Autodesk Inventor part; units mm, degrees
ref_plane "YZ Plane" through (0, 0, 0) normal (1, 0, 0) x (0, 1, 0)
ref_plane "XZ Plane" through (0, 0, 0) normal (0, 1, 0) x (-1, 0, 0)
ref_plane "XY Plane" through (0, 0, 0) normal (0, 0, 1) x (1, 0, 0)
sketch "Sketch1" plane through (0, 0, 0) normal (0, 0, 1) x (1, 0, 0)
  line L0 (0, 0) -> (3.8, 0)
  line L1 (3.8, 0) -> (3.8, 17) construction
  line L2 (3.8, 17) -> (0, 17)
  line L3 (0, 17) -> (0, 0) construction
  line L4 (3.8, 17) -> (3.8, 11.325)
  line L5 (3.8, 0) -> (3.8, 5.675)
  line L6 (3.8, 8.5) -> (16.8, 8.5) construction
  line L7 (16.8, 10.45) -> (16.8, 6.55) construction
  line L8 (3.8, 5.675) -> (18.8, 6.6846)
  line L9 (3.8, 11.325) -> (18.8, 10.3154)
  line L10 (18.8, 10.3154) -> (18.8, 6.6846)
  line L11 (0, 17) -> (0, 12)
  line L12 (0, 0) -> (0, 5)
  line L13 (0, 8.5) -> (-15, 8.5) construction
  line L14 (-15, 10.5) -> (-15, 6.5) construction
  line L15 (0, 12) -> (-16, 10.4)
  line L16 (0, 5) -> (-16, 6.6)
  line L17 (-16, 10.4) -> (-16, 6.6)
  dimension "d0" = 3.8
  dimension "d1" = 17
  dimension "d2" = 5.675
  dimension "d3" = 5.675
  dimension "d4" = 13
  dimension "d5" = 3.9
  dimension "d8" = 15
  dimension "d9" = 15
  dimension "d10" = 5
  dimension "d11" = 5
  dimension "d12" = 15
  dimension "d13" = 4
  dimension "d14" = 16
  dimension "d15" = 16
  dimension "d75" = 7.701
extrude "Horn_Body" add sketch "Sketch1" along normal blind 2
fillet "Fillet1" radius 1.9 4 edges at (3.8, 17, 1) (0, 17, 1) (0, 0, 1) (3.8, 0, 1)
fillet "Fillet2" radius 1.9 2 edges at (18.8, 6.6846, 1) (18.8, 10.3154, 1)
fillet "Fillet3" radius 2 2 edges at (-16, 10.4, 1) (-16, 6.6, 1)
sketch "Sketch2" plane through (0, 0, 0) normal (0, 0, -1) x (-1, 0, 0)
  circle A0 centre (-1.9, 8.5) radius 3.55
  line L0 (18.55, 8.5) -> (-27.4875, 8.5) construction
  line L1 (16, 8.59) -> (16, 8.41)
  line L2 (-1.9, 22.225) -> (-1.9, -4.7625) construction
  line L3 (-3.8, 11.325) -> (-3.8, 15.1)
  line L4 (0, 15.1) -> (0, 12)
  point P0 (0, 0)
  point P1 (16, 8.5)
  dimension "d21" = 7.1
  dimension "d22" = 3.8
  dimension "d23" = 1.9
extrude "Shaft_Connector" add sketch "Sketch2" along normal blind 2.7
sketch "Sketch3" plane through (1.9, 8.5, -2.7) normal (0, 0, -1) x (-1, 0, 0)
  circle A0 centre (0, 0) radius 2.25
  point P0 (1.9, -8.5)
  dimension "d26" = 4.5
extrude "Shaft_Opening" cut sketch "Sketch3" against normal blind 2
sketch "Sketch4" plane through (1.9, 8.5, -0.7) normal (0, 0, -1) x (-1, 0, 0)
  circle A0 centre (0, 0) radius 1.25
  point P0 (1.9, -8.5)
  dimension "d29" = 2.5
extrude "Opening_Horn_FixationScrew" cut sketch "Sketch4" against normal up to surface (2.7 mm away)
sketch "Sketch6" plane through (0, 0, 2) normal (0, 0, 1) x (1, 0, 0)
  line L0 (-18.55, 8.5) -> (21.1375, 8.5) construction
  line L1 (-16, 8.59) -> (-16, 8.41)
  line L2 (1.9, 19.05) -> (1.9, -2.3164) construction
  line L3 (3.8, 11.325) -> (3.8, 15.1)
  line L4 (0, 15.1) -> (0, 12)
  circle A0 centre (-11.1, 8.54) radius 0.25
  circle A1 centre (-9.1, 8.5) radius 0.25
  circle A2 centre (-7.1, 8.5) radius 0.25
  circle A3 centre (-3.1, 8.5) radius 0.25
  circle A4 centre (-5.1, 8.5) radius 0.25
  circle A5 centre (-13.1, 8.5) radius 0.25
  circle A6 centre (-15.1, 8.5) radius 0.25
  circle A7 centre (6.9, 8.5) radius 0.25
  circle A8 centre (8.9, 8.5) radius 0.25
  circle A9 centre (10.9, 8.5) radius 0.25
  circle A10 centre (12.9, 8.5) radius 0.25
  circle A11 centre (14.9, 8.5) radius 0.25
  circle A12 centre (16.9, 8.5) radius 0.25
  circle A13 centre (1.9, 13.5) radius 0.25
  circle A14 centre (1.9, 15.5) radius 0.25
  circle A15 centre (1.9, 3.5) radius 0.25
  circle A16 centre (1.9, 1.5) radius 0.25
  point P0 (0, 0)
  point P1 (-16, 8.5)
  dimension "d35" = 3.8
  dimension "d36" = 1.9
  dimension "d37" = 0.5
  dimension "d38" = 0.5
  dimension "d39" = 0.5
  dimension "d41" = 0.5
  dimension "d42" = 0.5
  dimension "d43" = 5
  dimension "d44" = 2
  dimension "d46" = 2
  dimension "d47" = 2
  dimension "d48" = 2
  dimension "d49" = 0.5
  dimension "d50" = 0.5
  dimension "d51" = 2
  dimension "d52" = 2
  dimension "d53" = 0.5
  dimension "d54" = 0.5
  dimension "d55" = 0.5
  dimension "d56" = 0.5
  dimension "d57" = 0.5
  dimension "d58" = 5
  dimension "d59" = 2
  dimension "d60" = 2
  dimension "d61" = 2
  dimension "d62" = 2
  dimension "d63" = 0.5
  dimension "d64" = 2
  dimension "d65" = 0.5
  dimension "d66" = 0.5
  dimension "d67" = 0.5
  dimension "d68" = 0.5
  dimension "d69" = 5
  dimension "d70" = 2
  dimension "d71" = 5
  dimension "d72" = 2
extrude "Connection_Holes" cut sketch "Sketch6" against normal up to surface (2 mm away)
sketch "Sketch8" plane through (0, 0, 2) normal (0, 0, 1) x (1, 0, 0)
  circle A0 centre (1.9, 8.5) radius 1.25
  circle A1 centre (1.9, 8.5) radius 2.5
  circle A2 centre (1.9, 8.5) radius 3.1
  point P0 (0, 0)
  dimension "d80" = 5
  dimension "d81" = 6.2
extrude "Centering_RIng" add sketch "Sketch8" along normal blind 1 contours A2
equation "\"d14\" = d15"
equation "\"d23\" = 0.5 * d22"
equation "\"d36\" = 0.5 * d35"
properties part number "Servo_Horn_Cross_TGY"
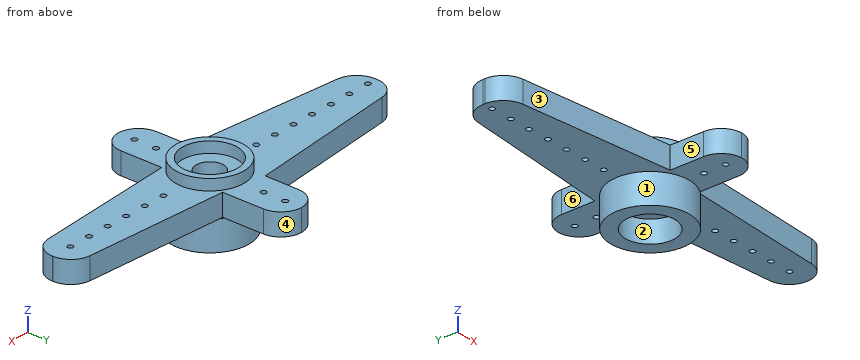
Geometry: final body of the model. Coordinates: model frame, mm. Face numbers are marked on the shaded views. A direction names the side the tool comes from. Coordinates: 2 decimals unless noted, no trailing zeros. Order: outer loops, then holes, each group sorted by start corner. A loop starts at its lowest first (then second) coordinate and runs counter-clockwise, first axis right, second up. Notation, with made-up numbers: (-34.5, 46) -> (1.5, 46) arc R35 ccw to (1.5, 78) -> close; hole circle Ø10 at (-24.5, 37.25). An arc over 180 degrees is marked (long way). Use CSV: the item, a comma, the result in double quotes.
1) Pin query (flat end, axial travel): pin 1 Ø5 at (x, y) = (1, 8) entering from -Z; pin 2 Ø1.6 at (y, z) = (13.5, 0.5) entering from -X; pin 3 Ø3 at (x, y) = (12, 7.5) entering from -Z; pin 4 Ø1 at (y, z) = (4.5, 1) entering from +X. Return the tip coordinate at first contact, or that it passes through.
Findings:
pin 1,"stops at z = -2.7"
pin 2,"stops at x = 0"
pin 3,"stops at z = 0"
pin 4,"stops at x = 3.8"
2) Line query: line 1 (Y direction, x = 1.9, z = 1.6); line 2 (Y direction, x = 16.9, z = 1); line 3 (Z direction, x = 4, y = 9.75). Output: solid intervals per line, ascending.
Findings:
line 1,"y = 0 to 1.25, 1.75 to 3.25, 3.75 to 7.25, 9.75 to 13.25, 13.75 to 15.25, 15.75 to 17"
line 2,"y = 6.56 to 8.25, 8.75 to 10.44"
line 3,"z = -2.7 to 2"
3) Access query for the marked faces 4, 5 and 6. Directions: +Z, -Z, +X, -X, +Y, -Y. A direction counts if a zero-diameter tool reaches every point of the face in a straight line with its end or side. Return the directions, or none.
Findings:
face 4,"+Z, -Z, +X, +Y"
face 5,"+Z, -Z, -X, -Y"
face 6,"+Z, -Z, -X, +Y"
4) Mould query, pull axis X, two halves, no side actions, for the marked faces 1, 2 and 3. Classes: +X half, -X half, draft (parallel to the pull), parting line (faces both ways), or undercut.
Findings:
face 1,"parting line"
face 2,"undercut"
face 3,"-X half"
5) Section C-C on x = 14. Output: boundary loops of the cut face in (y, z).
Findings:
outline,"(6.36, 0) -> (10.64, 0) -> (10.64, 2) -> (6.36, 2) -> close"
6) Section B-B on x = -4.5. Output: boundary loops of the cut face in (y, z), then the cut area to 3 significant figures.
Findings:
outline,"(5.45, 0) -> (11.55, 0) -> (11.55, 2) -> (5.45, 2) -> close"
area,"12.2 mm^2"
7) Section A-A on z = 0.9. State how many separate pieces and enclosed holes the cut face has, then the cut area to 3 significant figures.
Findings:
separate pieces,"1"
enclosed holes,"18"
area,"207 mm^2"
